Geometry check sheet. Reference: drawing and pictorial views, mm from the part's lowest x, y, z. A direction names the side the tool comes from. Give positions to 0.01 mm unless a question says otherwise; leave off trailing zeros. Write each loop counter-clockwise with the first axis right and the second up, starting at its lowest first coordinate (ties: lowest second). Pieces come first, ordered by that corner, then holes.
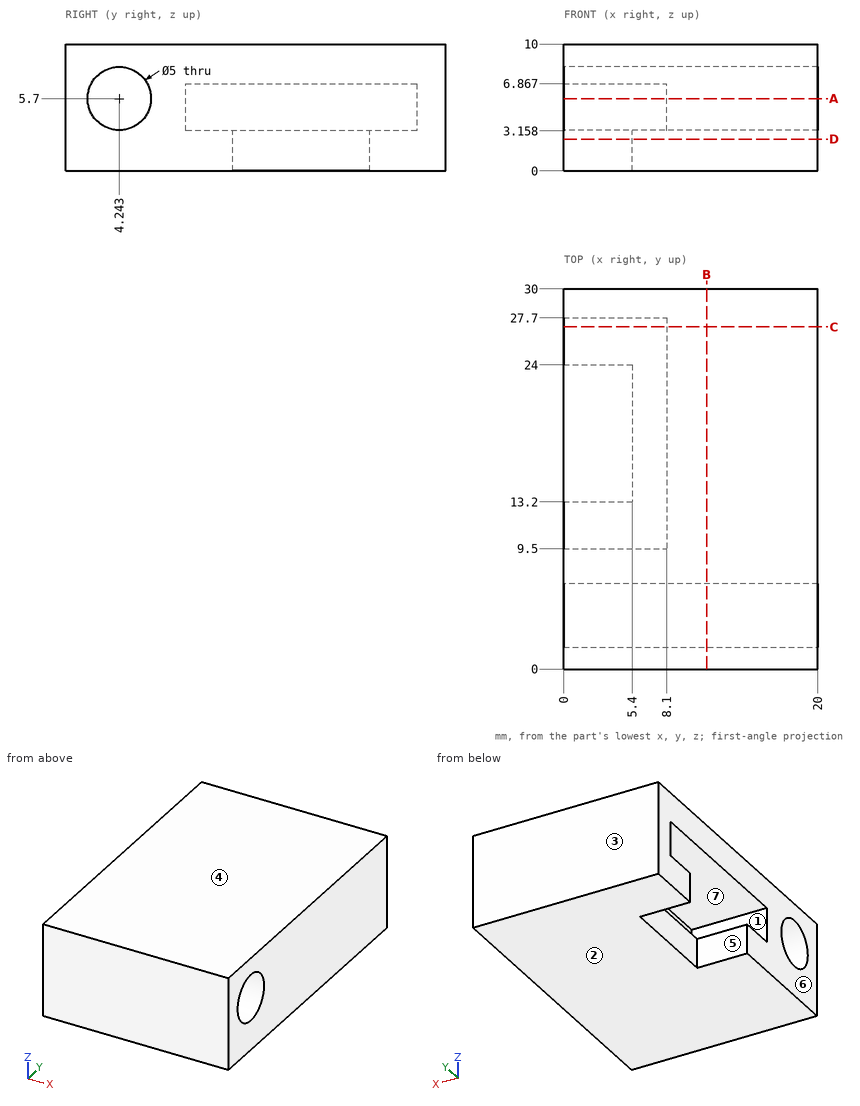
Item 1: Sectioned sample at B-B on x = 11.25. Record the cut outline in (y, z), then the cut area to 3 significant figures.
Answer key:
outline: (0, 0) - (30, 0) - (30, 10) - (0, 10) - close; hole circle Ø5 at (4.24, 5.7)
area: 280 mm2
Item 2: Scan lines: line 1 along Y through (x, z) = (1.25, 0.5); line 2 along Z through (x, y) = (4, 26.5); line 3 along Y through (x, z) = (14.5, 5.75). Record each from-to range of solid material in increasing order.
Answer key:
line 1: y = 0 to 13.2, 24 to 30
line 2: z = 0 to 3.16, 6.87 to 10
line 3: y = 0 to 1.74, 6.74 to 30
Item 3: Depth check by flat-ended pin: pin 1 (4 mm diameter, centred on x = 2.5, y = 21, fed in from -Z); pin 2 (0.9 mm diameter, centred on y = 21, z = 1, fed in from -X). Enter the tip coordinate at first touch or a pass-through.
Answer key:
pin 1: stops at z = 6.87
pin 2: stops at x = 5.4
Item 4: Sectioned sample at D-D on z = 2.5. Record the cut outline in (x, y).
Answer key:
outline: (0, 0) - (20, 0) - (20, 30) - (0, 30) - (0, 24) - (5.4, 24) - (5.4, 13.2) - (0, 13.2) - close
Item 5: Sectioned sample at A-A on z = 5.7. Record the cut outline in (x, y).
Answer key:
outline: (0, 0) - (20, 0) - (20, 1.74) - (0, 1.74) - close; (0, 6.74) - (20, 6.74) - (20, 30) - (0, 30) - (0, 27.7) - (8.1, 27.7) - (8.1, 9.5) - (0, 9.5) - close
Item 6: Sectioned sample at C-C on y = 27. Record the cut outline in (x, z).
Answer key:
outline: (0, 0) - (20, 0) - (20, 10) - (0, 10) - (0, 6.87) - (8.1, 6.87) - (8.1, 3.16) - (0, 3.16) - close
Item 7: Release check for a two-part mould opening along Z. For the marked faces 1, 2, 3 and 4 record: released by +Z, released by -Z, zero draft, split by the parting line, or undercut.
Answer key:
face 1: undercut
face 2: released by -Z
face 3: zero draft
face 4: released by +Z
Item 8: Set-up check for the marked faces 5, 6 and 7: record each of +Z, -Z, +X, -X, +Y, -Y from which the full face is reachable in a straight line by a thin tool's end or side.
Answer key:
face 5: -Z, -X
face 6: +Z, -Z, -X, +Y, -Y
face 7: -X
